Geometry check sheet. Reference: drawing and pictorial views, mm from the part's lowest x, y, z. Give positions to 0.01 mm unless a question says otherwise; leave off trailing zeros. Write each loop counter-clockwise with the first axis right and the second up, starting at its lowest first coordinate (ties: lowest second). Pieces come first, ordered by that corner, then holes. Notation, with made-up numbers: M -11.75,15.25 L 40.25,15.25 A27 cw 40.25,35.25 Z; hole C 34,-32.75 d3. An arc over 180 degrees is marked long. Write item = value, one per line. Start each with the question number.
1) Cross-section at D-D, the plane x = 10. Record the cut outline in (y, z), plus the area to 4 significant figures.
2) Scan lines: line 1 along Z through (x, y) = (10, 1.7); line 2 along Z through (x, y) = (90, 3.65); line 3 along Z through (x, y) = (86, 0.95). Record each from-to range of solid material in increasing order. Write a range as [from, to].
3) Cross-section at C-C, the plane y = 3.4. Record the cut outline in (x, z).
4) Cross-section at A-A, the plane z = 10. Record the cut outline in (x, y).
5) Go/stop test with a flat-tipped pin: pin 1 (4.5 mm diameter, centred on x = 10, z = 10, fed in from +Y). Record where the tip stops, or that it passes through.
6) Cross-section at B-B, the plane x = 90. Record the cut outline in (y, z).
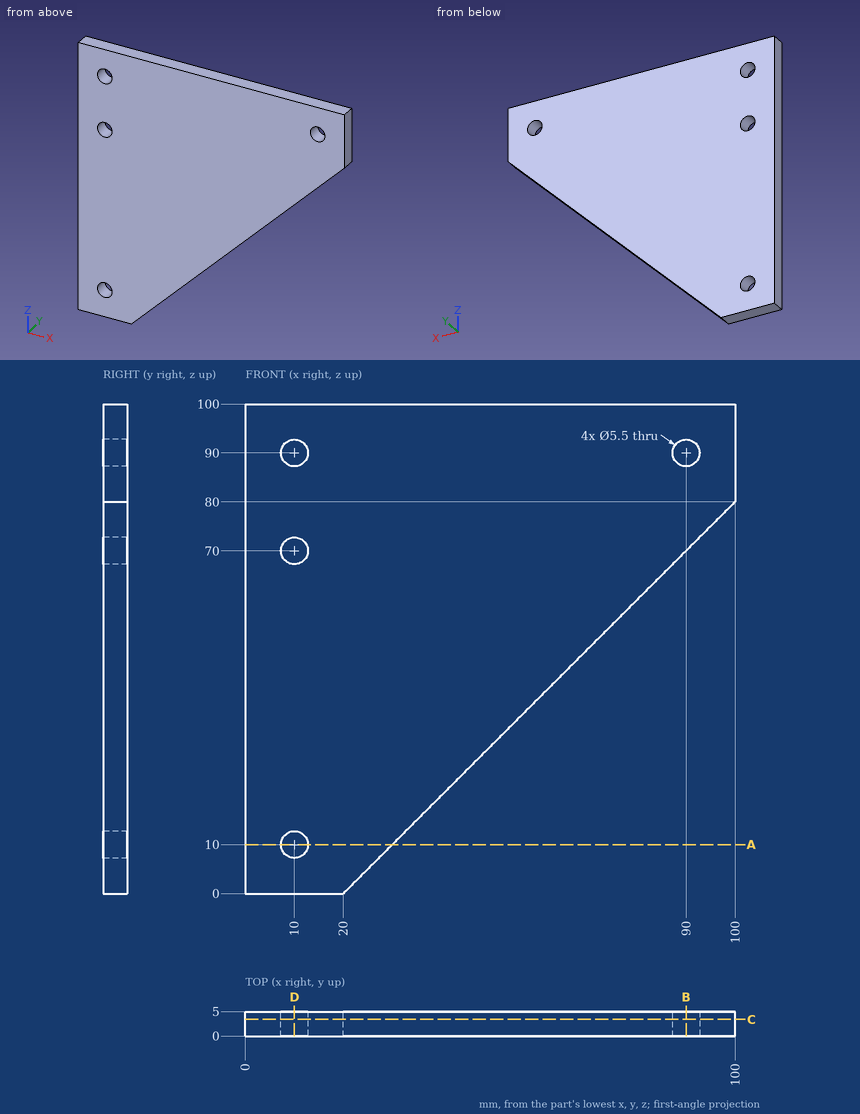
Reply:
q1.outline = M 0,0 L 5,0 L 5,7.25 L 0,7.25 Z; M 0,12.75 L 5,12.75 L 5,67.25 L 0,67.25 Z; M 0,72.75 L 5,72.75 L 5,87.25 L 0,87.25 Z; M 0,92.75 L 5,92.75 L 5,100 L 0,100 Z
q1.area = 417.5 mm2
q2.line_1 = [0, 7.25], [12.75, 67.25], [72.75, 87.25], [92.75, 100]
q2.line_2 = [70, 87.25], [92.75, 100]
q2.line_3 = [66, 100]
q3.outline = M 0,0 L 20,0 L 100,80 L 100,100 L 0,100 Z; hole C 10,10 d5.5; hole C 10,70 d5.5; hole C 10,90 d5.5; hole C 90,90 d5.5
q4.outline = M 0,0 L 7.25,0 L 7.25,5 L 0,5 Z; M 12.75,0 L 30,0 L 30,5 L 12.75,5 Z
q5.pin_1 = through
q6.outline = M 0,70 L 5,70 L 5,87.25 L 0,87.25 Z; M 0,92.75 L 5,92.75 L 5,100 L 0,100 Z
